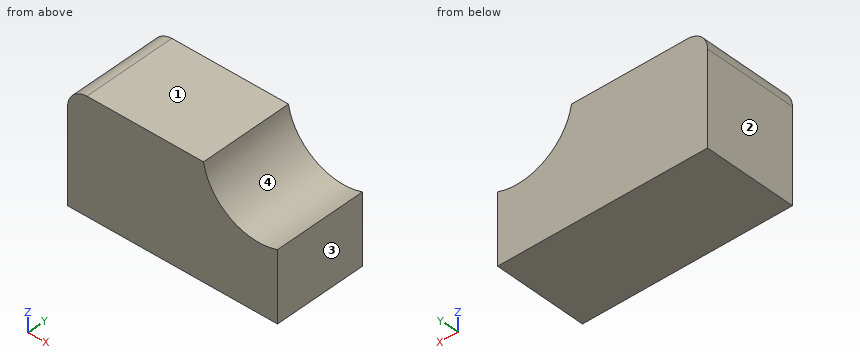
from build123d import *

# Parameters (mm, degrees)
F1_DEPTH = 25.4


with BuildPart() as f1:
    # F0 (on Front) → F1 (new body)
    with BuildSketch(Plane.XZ):
        with BuildLine():
            Line((2.19345, 25.4), (2.19345, 0))
            Line((2.19345, 0), (59.34345, 0))
            Line((59.34345, 0), (59.34345, 19.05))
            ThreePointArc((59.34345, 19.05), (46.513424, 20.262757), (39.207902, 30.87924))
            Line((39.207902, 30.87924), (7.457902, 30.87924))
            ThreePointArc((7.457902, 30.87924), (3.722837, 29.199227), (2.19345, 25.4))
        make_face()
    extrude(amount=F1_DEPTH)


solid = f1.part
Source: CAD feature listing. Evaluate the final solid. Frame: model axes, mm. Face numbers are marked on the shaded views. Round coordinates to 2 decimals unless told otherwise and drop trailing zeros. Loops run counter-clockwise (first coordinate to the right, second up) from the corner with the lowest first, then second, coordinate; pieces in that order, holes last. Notation, with made-up numbers: (75.5, -16) - (101.5, -16) arc R22 ccw to (101.5, -5) - close; hole circle Ø6 at (10, 7.5). An arc over 180 degrees is marked (long way). Write item = value, one per line. Start each with the question number.
(1) Pin query (flat end, axial travel): pin 1 (2 mm diameter, centred on x = 44.5, y = -18.5, fed in from +Z). Return the tip coordinate at first contact, or that it passes through.
(2) Section query A-A, the plane y = -17.5. Output: boundary loops of the cut face in (x, z).
(3) Section query B-B, the plane z = 26. Output: boundary loops of the cut face in (x, y).
(4) Pull-direction query (X, two-part tool) for the marked faces 1, 2, 3 and 4; classes: +X half, -X half, draft (parallel to the pull), parting line (faces both ways), or undercut.
(5) Ray query, line 1 along X through (y, z) = (-8.25, 26); line 2 along Z through (x, y) = (45.5, -1.25); line 3 along Z through (x, y) = (42.5, -14.5). Return the intervals inside material, ascending. Write a range as from..to.
(6) Section query C-C, the plane x = 52.5. Output: boundary loops of the cut face in (y, z), plus the area to 3 significant figures.
Conclusion:
q1.pin_1 = 22.58
q2.outline = (2.19, 0) - (59.34, 0) - (59.34, 19.05) arc R15.23 cw to (39.21, 30.88) - (7.46, 30.88) arc R5.48 ccw to (2.19, 25.4) - close
q3.outline = (2.23, -25.4) - (40.91, -25.4) - (40.91, 0) - (2.23, 0) - close
q4.face_1 = draft
q4.face_2 = -X half
q4.face_3 = +X half
q4.face_4 = undercut
q5.line_1 = 2.23..40.91
q5.line_2 = 0..20.91
q5.line_3 = 0..23.68
q6.outline = (-25.4, 0) - (0, 0) - (0, 18.26) - (-25.4, 18.26) - close
q6.area = 464 mm2
